Can you work these out from the model? Positions are in its coordinate system, mm. A direction names the side the tool comes from. Give positions to 0.01 mm unless a question says otherwise; leave off trailing zeros. Order: outer loops, then holes, each group sorted by start corner. A loop starts at its lowest first (then second) coordinate and runs counter-clockwise, first axis right, second up. Notation, with made-up numbers: M 66.5,78.5 L 106.5,78.5 A18 ccw 106.5,99.5 Z; hole C -37.5,35.25 d10. An arc over 180 degrees is marked long. Answer as a JSON object with one key per item and string values.
```python
from build123d import *

# Parameters (mm, degrees)
ESQUISSE2_R        = 4.5
BOSS_EXTRU_1_DEPTH = 20
CHANFREIN1_SIZE    = 0.5
ESQUISSE3_R        = 3
BOSS_EXTRU_4_DEPTH = 0.1
ESQUISSE5_R        = 0.75
BOSS_EXTRU_5_DEPTH = 20


with BuildPart() as part:
    # Esquisse2 → Boss.-Extru.1 (new body)
    with BuildSketch(Plane.XY):
        Circle(ESQUISSE2_R)
    extrude(amount=BOSS_EXTRU_1_DEPTH)

    # Chanfrein1
    chanfrein1_edges = [part.edges().sort_by_distance(p)[0] for p in [
        (-4.5, 0, 0),
        (-4.5, 0, 20),
    ]]
    chamfer(chanfrein1_edges, length=CHANFREIN1_SIZE)

    # Esquisse3 → Boss.-Extru.4 (add)
    with BuildSketch(Plane.XY.offset(20)):
        Circle(ESQUISSE3_R)
    extrude(amount=BOSS_EXTRU_4_DEPTH)

    # Esquisse5 → Boss.-Extru.5 (add)
    with BuildSketch(Plane(origin=(0, 0, 0), x_dir=(-1, 0, 0), z_dir=(0, 0, -1))):
        with Locations(Location((0.76, 0, 0), (0, 0, 180))):
            Circle(ESQUISSE5_R)
        with Locations(Location((-0.76, 0, 0), (0, 0, 180))):
            Circle(ESQUISSE5_R)
    extrude(amount=BOSS_EXTRU_5_DEPTH)


solid = part.part
```
1) I want a section at C-C on z = 10.5. Write out the boundary of the cut face in (x, y).
Results found:
{"outline": "C 0,0 d9"}
2) I need wall thicknesses on L1, parallel to Z at x = 2.5, y = 3; L2, parallel to Z at x = 0.5, y = -2; L3, parallel to X at y = -0.5, z = -3. Which ranges of each line are inside material? Lowest first, please.
Results found:
{"L1": "z = 0 to 20", "L2": "z = 0 to 20.1", "L3": "x = -1.32 to -0.2, 0.2 to 1.32"}
3) For faces 1 (the face through (1, 3, 20)), 2 (the face through (-1, 0, -20)), which set-ups out of +Z, -Z, +X, -X, +Y, -Y let a thin tool reach every point of the face, with its end or its side?
Results found:
{"face 1": "+Z", "face 2": "-Z, +X, -X, +Y, -Y"}
4) I want a section at A-A on z = -8.5. Write out the boundary of the cut face in (x, y).
Results found:
{"outline": "C -0.76,0 d1.5; C 0.76,0 d1.5"}
5) I'm going to push flat-ended pins straight in: pin 1 Ø3 at (y, z) = (2.5, 11.5) entering from +X; pin 2 Ø3 at (x, z) = (-0.5, 15.5) entering from -Y; pin 3 Ø4 at (y, z) = (1.5, -8) entering from +X; pin 4 Ø1 at (x, z) = (1.5, 4) entering from +Y. Where does each tip first touch, or does it pass through?
Results found:
{"pin 1": "stops at x = 4.39", "pin 2": "stops at y = -4.5", "pin 3": "stops at x = 1.51", "pin 4": "stops at y = 4.39"}
6) Thinking about a two-plate mould opening in X: for faces 3 (the face through (-0.59, 4.46, 9.87)), 4 (the face through (1, 0, -20)), 5 (the face through (-1.51, -0.03, -9.86)), which applies, pulls with the +X half, pulls with the -X half, needs draft (parallel to the pull), parting line crosses it, or undercut?
Results found:
{"face 3": "parting line crosses it", "face 4": "needs draft", "face 5": "undercut"}
